Answer from the drawing. Dimensions are ordinates in mm from the lowest x, y and z of the part. Coordinates: 2 decimals unless noted, no trailing zeros. Write each loop counter-clockwise with the first axis right and the second up, starting at its lowest first coordinate (ties: lowest second). Pieces come first, ordered by that corner, then holes. Notation, with made-up numbers: (87, 14.25) -> (115, 14.25) arc R28 cw to (115, 50.25) -> close; hole circle Ø10 at (81, 21.5). An arc over 180 degrees is marked (long way). Return JSON: item names as keys, results as strings.
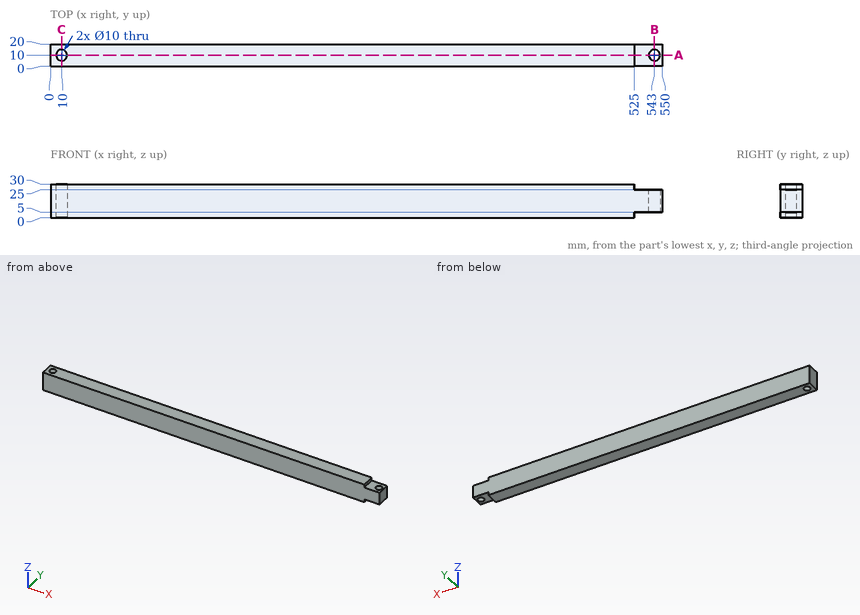
1. The part is cut by section C-C (x = 10). Determine the outline of the cut face in (y, z).
Taken from the geometry:
{"outline": "(0, 0) -> (5, 0) -> (5, 30) -> (0, 30) -> close; (15, 0) -> (20, 0) -> (20, 30) -> (15, 30) -> close"}
2. Consider L1, parallel to Y at x = 543, z = 20.25; L2, parallel to X at y = 8.75, z = 9; L3, parallel to X at y = 4.5, z = 4.25. Determine where each line is inside the solid, lowest interval first.
Taken from the geometry:
{"L1": "y = 0 to 5, 15 to 20", "L2": "x = 0 to 5.16, 14.84 to 538.16, 547.84 to 550", "L3": "x = 0 to 525"}
3. The part is cut by section B-B (x = 543). Determine the outline of the cut face in (y, z).
Taken from the geometry:
{"outline": "(0, 5) -> (5, 5) -> (5, 25) -> (0, 25) -> close; (15, 5) -> (20, 5) -> (20, 25) -> (15, 25) -> close"}
4. The part is cut by section A-A (y = 10). Determine the outline of the cut face in (x, z).
Taken from the geometry:
{"outline": "(0, 0) -> (5, 0) -> (5, 30) -> (0, 30) -> close; (15, 0) -> (525, 0) -> (525, 5) -> (538, 5) -> (538, 25) -> (525, 25) -> (525, 30) -> (15, 30) -> close; (548, 5) -> (550, 5) -> (550, 25) -> (548, 25) -> close"}
5. Flat-ended cylindrical pins translate along their axes: pin 1 Ø2.5 at (y, z) = (8.5, 28.5) entering from +X; pin 2 Ø10 at (x, y) = (535, 6.5) entering from -Z; pin 3 Ø8 at (x, y) = (543, 10) entering from -Z. Find the tip coordinate at first contact, or state that the pin passes through.
Taken from the geometry:
{"pin 1": "stops at x = 525", "pin 2": "stops at z = 5", "pin 3": "passes through"}
